The model under review builds one solid part; all positions refer to its coordinate system, in mm. A direction names the side the tool comes from. Round coordinates to 2 decimals unless told otherwise and drop trailing zeros. Loops run counter-clockwise (first coordinate to the right, second up) from the corner with the lowest first, then second, coordinate; pieces in that order, holes last. Notation, with made-up numbers: (4, 88.5) -> (17, 88.5) arc R25 ccw to (17, 117.5) -> close; hole circle Ø5 at (41, -20). An arc over 180 degrees is marked (long way). Use a Markdown table: item, result. Add a question column.
1) Consider section C-C on y = 31. Give the boundary of the cut face in (x, z), plus the area to 3 significant figures.
2) Insertion check: pin 1 (4 mm diameter, centred on x = 36.5, y = 55.5, fed in from +Z); pin 2 (0.8 mm diameter, centred on x = 19, z = -1.5, fed in from +Y); pin 3 (1 mm diameter, centred on y = 3, z = 7, fed in from +X); pin 4 (1.8 mm diameter, centred on x = 22, y = 3.5, fed in from +Z). Each pin has a flat end and moves straight along its axis. Give the tip position at first contact, or say it passes through.
3) Wall thickness on probe 1 along Y at (x, z) = (4.5, 7.5); probe 2 along Y at (x, z) = (15.5, 9.5); probe 3 along Z at (x, y) = (39.5, 29): over which ranges is each line inside the solid? List them lowest first.
4) Consider section A-A on z = 2.25. Give the boundary of the cut face in (x, y), plus the area to 3 significant figures.
5) For faces 4 (the flat face through (24.65, 9.644, 4.694)), 5 (the flat face through (25, -2, 11.203)), 6 (the flat face through (24.65, 25.523, 4.979)), list the 3-axis set-ups (+Z, -Z, +X, -X, +Y, -Y) from which the entire face can be reached by the end or side of a thin tool; tool diameter is ignored.
6) Mouldability with a two-part tool opening along Y and no side actions: class faces 1 (the flat face through (50, 29, -3)), 2 (the cylindrical face through (25.35, -5.32, 10.63)), 3 (the flat face through (24.65, 33.904, -0.936)) as released by +Y, released by -Y, zero draft, split by the parting line, or undercut.
Autodesk Fusion 360 part; units mm, degrees
sketch "Sketch1" plane through (0, 0, 0) normal (1, 0, 0) x (0, 1, 0)
  line L0 (0, 0) -> (9.7495, 79.4037)
  line L1 (9.7495, 79.4037) -> (18.6825, 78.3069)
  line L2 (18.6825, 78.3069) -> (8.9329, -1.0968)
  line L3 (8.9329, -1.0968) -> (0, 0)
  line L4 (1.5446, -0.1007) -> (5.0446, -0.1007)
  line L5 (5.0446, -0.1007) -> (5.0446, -2.1007)
  line L6 (5.0446, -2.1007) -> (1.5446, -2.1007)
  line L7 (1.5446, -2.1007) -> (1.5446, -0.1007)
  line L8 (0, 140) -> (0, -50)
  line L9 (25, 0) -> (33.3623, 79.5618)
  line L10 (33.3623, 79.5618) -> (43.3075, 78.5165)
  line L11 (43.3075, 78.5165) -> (34.9452, -1.0453)
  line L12 (34.9452, -1.0453) -> (25, 0)
  line L13 (-90, 0) -> (150, 0)
  line L14 (28.2277, -2.2181) -> (31.7277, -2.2181)
  line L15 (31.7277, -2.2181) -> (31.7277, -0.2181)
  line L16 (31.7277, -0.2181) -> (28.2277, -0.2181)
  line L17 (28.2277, -0.2181) -> (28.2277, -2.2181)
  dimension "d1" = 80
  dimension "d2" = 9
  dimension "d9" = 3.5
  dimension "d10" = 2
  dimension "d12" = 80
  dimension "d13" = 10
  dimension "d15" = 97
  dimension "d16" = 96
  dimension "d17" = 25
  dimension "d18" = 3.5
  dimension "d19" = 2
sketch "Sketch2" plane through (0, 0, 0) normal (1, 0, 0) x (0, 1, 0)
  line L0 (-5.92, 11.2031) -> (64.08, 11.2031)
  line L1 (64.08, 11.2031) -> (64.08, -8.7969)
  line L2 (64.08, -8.7969) -> (-5.92, -8.7969)
  line L3 (-5.92, -8.7969) -> (-5.92, 11.2031)
  dimension "d3" = 70
  dimension "d4" = 20
extrude "Extrude1" add sketch "Sketch2" along normal blind 50
extrude "Extrude2" cut sketch "Sketch1" along normal blind 50
fillet "Fillet1" radius 1 4 edges at (25, 5.0446, -0.6194) (25, 1.5446, -0.1897) (25, 31.7277, -0.7071) (25, 28.2277, -0.3392)
fillet "Fillet2" radius 1 4 edges at (25, 10.4432, 11.2031) (25, 36.2326, 11.2031) (25, 26.1775, 11.2031) (25, 1.3756, 11.2031)
fillet "Fillet3" radius 2 1 edges at (25, -5.92, 11.2031)
fillet "Fillet4" radius 17 1 edges at (25, 64.08, 11.2031)
Result set:
| question | item | result |
|---|---|---|
| 1 | outline | (0, -8.8) -> (50, -8.8) -> (50, -2.22) -> (0, -2.22) -> close |
| 1 | area | 329 mm2 |
| 2 | pin 1 | z = 9.94 |
| 2 | pin 2 | y = 63.63 |
| 2 | pin 3 | through |
| 2 | pin 4 | z = -2.1 |
| 3 | probe 1 | -5.92 to 0.92, 9.99 to 25.79, 35.84 to 57.67 |
| 3 | probe 2 | -5.9 to 1.17, 10.23 to 26, 36.05 to 54.5 |
| 3 | probe 3 | -8.8 to -2.22 |
| 4 | outline | (0, -5.92) -> (50, -5.92) -> (50, 0.28) -> (0, 0.28) -> close; (0, 9.34) -> (50, 9.34) -> (50, 25.24) -> (0, 25.24) -> close; (0, 35.29) -> (50, 35.29) -> (50, 62.05) -> (0, 62.05) -> close |
| 4 | area | 2,440 mm2 |
| 5 | face 4 | +Z, +X, -X |
| 5 | face 5 | +Z, +X, -X, +Y, -Y |
| 5 | face 6 | +X, -X |
| 6 | face 1 | zero draft |
| 6 | face 2 | released by -Y |
| 6 | face 3 | undercut |
